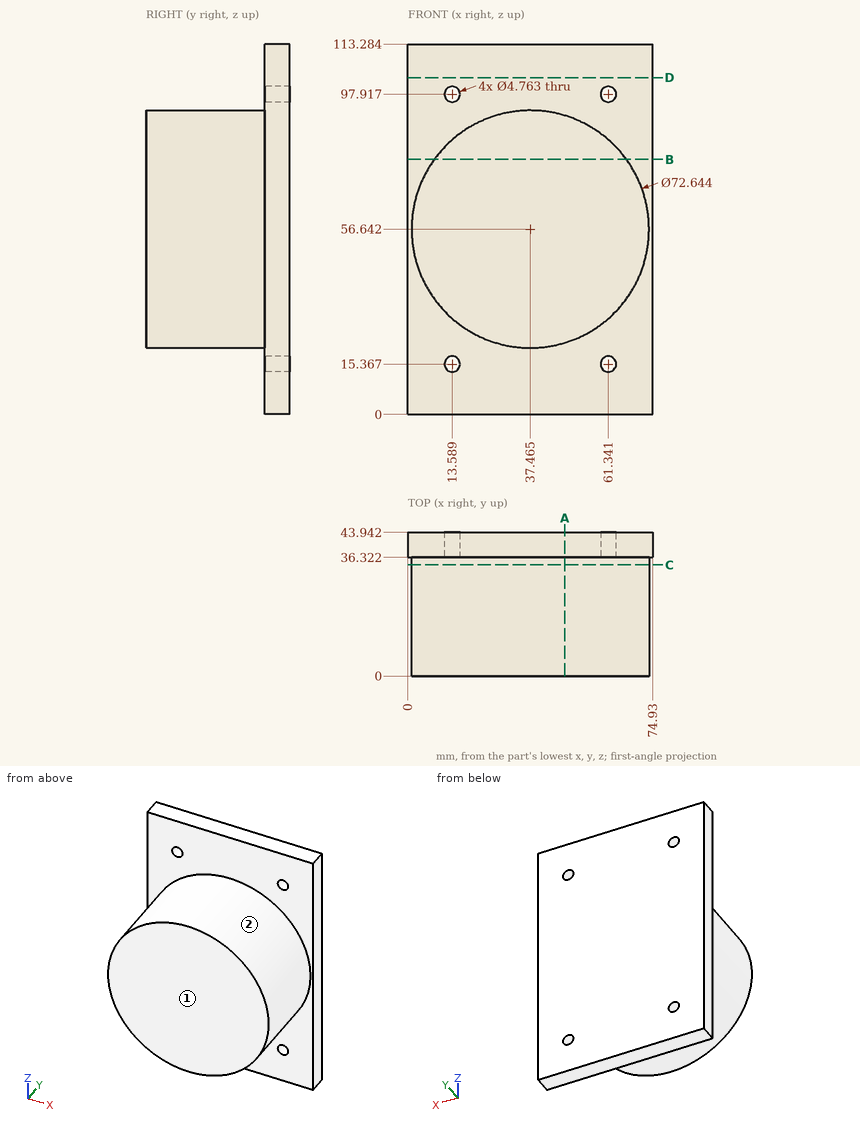
Can you work these out from the drawing? Everything is in mm from the part's minimum corner. A direction names the side the tool comes from. Coordinates: 2 decimals unless noted, no trailing zeros. Loops run counter-clockwise (first coordinate to the right, second up) from the corner with the lowest first, then second, coordinate; pieces in that order, holes last. Notation, with made-up numbers: (23.25, -9) - (51.25, -9) arc R21 ccw to (51.25, 30) - close; hole circle Ø8 at (9.5, 51.5). An arc over 180 degrees is marked (long way). Put each result on its own line as item: value. Start each with the question number.
Item 1: Suppose I cut it at C-C (y = 34). Please give me the cut outline in (x, z) (1 decimal).
Item 2: Which directions (+Z, -Z, +X, -X, +Y, -Y) give clear straight access to the entire face, cutting with the end or side of a thin tool? Please do the marked faces 1 and 2.
Item 3: Suppose I cut it at D-D (z = 103). Please give me the cut outline in (x, y).
Item 4: Suppose I cut it at A-A (x = 48). Please give me the cut outline in (y, z) (1 decimal), and give its area (3 significant figures).
Item 5: If I drill on line 1 along Y through (x, z) = (33, 109); line 2 along Z through (x, y) = (38, 13); line 3 along X through (y, z) = (19, 50) (1 decimal), over which ranges is the centre line in solid material (lowest first)?
Item 6: For pin 1 (1 mm diameter, centred on x = 16.5, y = 21.5, fed in from -Z) (1 decimal); pin 2 (5 mm diameter, centred on y = 12, z = 23.5, fed in from +X) (1 decimal); pin 3 (6 mm diameter, centred on x = 28.5, y = 27.5, fed in from -Z), each with a flat end and sliding along its axis, tell me the tip position at first contact or that it passes through.
Item 7: Suppose I cut it at B-B (z = 78). Please give me the cut outline in (x, y), and give its area (4 significant figures).
Here are the results:
1. outline: circle Ø72.6 at (37.5, 56.6)
2. face 1: +Z, -Z, +X, -X, -Y
2. face 2: -Y
3. outline: (0, 36.32) - (74.93, 36.32) - (74.93, 43.94) - (0, 43.94) - close
4. outline: (0, 21.9) - (36.3, 21.9) - (36.3, 0) - (43.9, 0) - (43.9, 113.3) - (36.3, 113.3) - (36.3, 91.4) - (0, 91.4) - close
4. area: 3,390 mm²
5. line 1: 36.32 to 43.94
5. line 2: 20.32 to 92.96
5. line 3: 1.8 to 73.2
6. pin 1: z = 26.6
6. pin 2: x = 57
6. pin 3: z = 20.81
7. outline: (0, 36.32) - (8.09, 36.32) - (8.09, 0) - (66.84, 0) - (66.84, 36.32) - (74.93, 36.32) - (74.93, 43.94) - (0, 43.94) - close
7. area: 2,705 mm²
